```python
from build123d import *

# Parameters (mm, degrees)
SKETCH_1_W          = 30
SKETCH_1_H          = 30
SKETCH_1_W_2        = 26
SKETCH_1_H_2        = 26
EXTRUDE_1_DEPTH     = 580
SKETCH_2_W          = 50
SKETCH_2_H          = 20
CUT_EXTRUDE_1_DEPTH = 581.969018107
SKETCH_3_R          = 2.1
CUT_EXTRUDE_2_DEPTH = 581.969018107
SKETCH_4_R          = 2.1
CUT_EXTRUDE_3_DEPTH = 581.969018107
SKETCH_7_R          = 1.65
CUT_EXTRUDE_6_DEPTH = 581.969018107
SKETCH_8_R          = 1.65
CUT_EXTRUDE_7_DEPTH = 581.969018107
SKETCH_9_R          = 1.65
CUT_EXTRUDE_8_DEPTH = 581.969018107


with BuildPart() as part:
    # 草图1 → 凸台-拉伸1 (new body)
    with BuildSketch(Plane.XY):
        Rectangle(SKETCH_1_W, SKETCH_1_H)
        Rectangle(SKETCH_1_W_2, SKETCH_1_H_2, mode=Mode.SUBTRACT)
    extrude(amount=EXTRUDE_1_DEPTH)

    # 草图2 → 切除-拉伸1 (cut, through all)
    with BuildSketch(Plane.ZY.offset(15)):
        with Locations((115, 0)):
            Rectangle(SKETCH_2_W, SKETCH_2_H)
        with Locations((465, 0)):
            Rectangle(SKETCH_2_W, SKETCH_2_H)
    extrude(amount=-CUT_EXTRUDE_1_DEPTH, mode=Mode.SUBTRACT)

    # 草图3 → 切除-拉伸2 (cut, through all)
    with BuildSketch(Plane(origin=(0, 15, 0), x_dir=(1, 0, 0), z_dir=(0, 1, 0))):
        with Locations(Location((7.5, -10, 0), (0, 0, 270))):
            Circle(SKETCH_3_R)
        with Locations(Location((-7.5, -10, 0), (0, 0, 270))):
            Circle(SKETCH_3_R)
        with Locations(Location((-7.5, -570, 0), (0, 0, 270))):
            Circle(SKETCH_3_R)
        with Locations(Location((7.5, -570, 0), (0, 0, 270))):
            Circle(SKETCH_3_R)
    extrude(amount=-CUT_EXTRUDE_2_DEPTH, mode=Mode.SUBTRACT)

    # 草图4 → 切除-拉伸3 (cut, through all)
    with BuildSketch(Plane(origin=(0, 15, 0), x_dir=(1, 0, 0), z_dir=(0, 1, 0))):
        with Locations(Location((7.5, -401.567476668, 0), (0, 0, 270))):
            Circle(SKETCH_4_R)
        with Locations(Location((-7.5, -401.567476668, 0), (0, 0, 270))):
            Circle(SKETCH_4_R)
        with Locations(Location((-7.5, -381.567476668, 0), (0, 0, 270))):
            Circle(SKETCH_4_R)
        with Locations(Location((7.5, -381.567476668, 0), (0, 0, 270))):
            Circle(SKETCH_4_R)
        with Locations(Location((7.5, -178.432523332, 0), (0, 0, 270))):
            Circle(SKETCH_4_R)
        with Locations(Location((-7.5, -178.432523332, 0), (0, 0, 270))):
            Circle(SKETCH_4_R)
        with Locations(Location((-7.5, -198.432523332, 0), (0, 0, 270))):
            Circle(SKETCH_4_R)
        with Locations(Location((7.5, -198.432523332, 0), (0, 0, 270))):
            Circle(SKETCH_4_R)
        with Locations((162.5, -178.432523332)):
            Circle(SKETCH_4_R)
        with Locations((177.5, -178.432523332)):
            Circle(SKETCH_4_R)
        with Locations((177.5, -198.432523332)):
            Circle(SKETCH_4_R)
        with Locations((162.5, -198.432523332)):
            Circle(SKETCH_4_R)
        with Locations((162.5, -381.567476668)):
            Circle(SKETCH_4_R)
        with Locations((162.5, -401.567476668)):
            Circle(SKETCH_4_R)
        with Locations((177.5, -401.567476668)):
            Circle(SKETCH_4_R)
        with Locations((177.5, -381.567476668)):
            Circle(SKETCH_4_R)
    extrude(amount=-CUT_EXTRUDE_3_DEPTH, mode=Mode.SUBTRACT)

    # 草图7 → 切除-拉伸6 (cut, through all)
    with BuildSketch(Plane(origin=(0, 15, 0), x_dir=(1, 0, 0), z_dir=(0, 1, 0))):
        with Locations(Location((0, -33.5, 0), (0, 0, 270))):
            Circle(SKETCH_7_R)
        with Locations(Location((0, -58.5, 0), (0, 0, 270))):
            Circle(SKETCH_7_R)
        with Locations((167, -73.072466057)):
            Circle(SKETCH_7_R)
        with Locations((167, -48.072466057)):
            Circle(SKETCH_7_R)
    extrude(amount=-CUT_EXTRUDE_6_DEPTH, mode=Mode.SUBTRACT)

    # 草图8 → 切除-拉伸7 (cut, through all)
    with BuildSketch(Plane(origin=(0, 15, 0), x_dir=(1, 0, 0), z_dir=(0, 1, 0))):
        with Locations(Location((3, -506.927533943, 0), (0, 0, 270))):
            Circle(SKETCH_8_R)
        with Locations(Location((7, -521.975679885, 0), (0, 0, 270))):
            Circle(SKETCH_8_R)
        with Locations(Location((3, -531.927533943, 0), (0, 0, 270))):
            Circle(SKETCH_8_R)
        with Locations(Location((7, -546.975679885, 0), (0, 0, 270))):
            Circle(SKETCH_8_R)
    extrude(amount=-CUT_EXTRUDE_7_DEPTH, mode=Mode.SUBTRACT)

    # 草图9 → 切除-拉伸8 (cut, through all)
    with BuildSketch(Plane(origin=(0, 15, 0), x_dir=(1, 0, 0), z_dir=(0, 1, 0))):
        with Locations(Location((-7.5, -445, 0), (0, 0, 270))):
            Circle(SKETCH_9_R)
        with Locations(Location((7.5, -445, 0), (0, 0, 270))):
            Circle(SKETCH_9_R)
        with Locations(Location((7.5, -485, 0), (0, 0, 270))):
            Circle(SKETCH_9_R)
        with Locations(Location((-7.5, -485, 0), (0, 0, 270))):
            Circle(SKETCH_9_R)
        with Locations(Location((-7.5, -95, 0), (0, 0, 270))):
            Circle(SKETCH_9_R)
        with Locations(Location((7.5, -95, 0), (0, 0, 270))):
            Circle(SKETCH_9_R)
        with Locations(Location((-7.5, -135, 0), (0, 0, 270))):
            Circle(SKETCH_9_R)
        with Locations(Location((7.5, -135, 0), (0, 0, 270))):
            Circle(SKETCH_9_R)
    extrude(amount=-CUT_EXTRUDE_8_DEPTH, mode=Mode.SUBTRACT)


solid = part.part
```
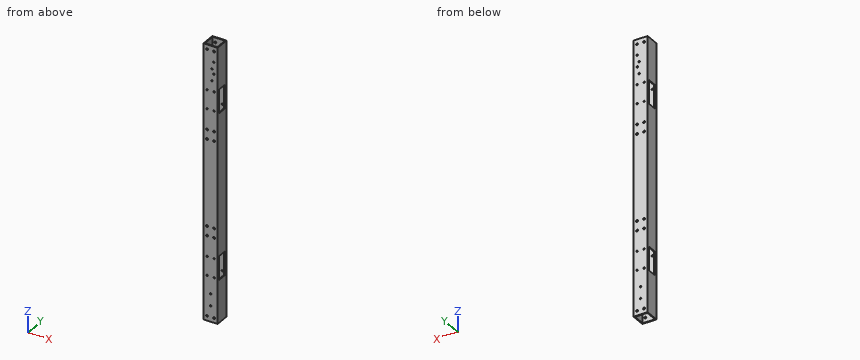
Part model, mm, in its own coordinate system. Round coordinates to 2 decimals unless told otherwise and drop trailing zeros. Write each loop counter-clockwise with the first axis right and the second up, starting at its lowest first coordinate (ties: lowest second). Pieces come first, ordered by that corner, then holes. Notation, with made-up numbers: (-15.5, 31) -> (-5.5, 31) arc R12 cw to (-5.5, 47) -> close; hole circle Ø6 at (89.25, 71.25). An arc over 180 degrees is marked (long way). Return JSON: item names as keys, results as strings. Group by question number.
Q1. Saw through at C-C on z = 351. Write the cut outline in (x, y), plus the area to 3 significant figures.
Q2. Saw through at A-A on z = 127. Write the cut outline in (x, y), plus the area to 3 significant figures.
Q3. Probe L1, parallel to X at y = -13.55, z = 95; L2, parallel to X at y = 11.5, z = 220. List the from-to ranges inside material, lowest first. Write a range as [from, to].
Q4. Pin check, flat tip, straight feed: pin 1 (3 mm diameter, centred on x = 7, z = 546.98, fed in from +Y). Stop position of the tip, or through.
Q5. Saw through at B-B on y = -1.25. Write the cut outline in (x, z), plus the area to 3 significant figures.
Answer:
{
 "1": {"outline": "(-15, -15) -> (15, -15) -> (15, 15) -> (-15, 15) -> close; hole (-13, -13) -> (13, -13) -> (13, 13) -> (-13, 13) -> close", "area": "224 mm2"},
 "2": {"outline": "(-15, -15) -> (15, -15) -> (15, -10) -> (13, -10) -> (13, -13) -> (-13, -13) -> (-13, -10) -> (-15, -10) -> close; (-15, 10) -> (-13, 10) -> (-13, 13) -> (13, 13) -> (13, 10) -> (15, 10) -> (15, 15) -> (-15, 15) -> close", "area": "144 mm2"},
 "3": {"L1": "[-15, -9.15], [-5.85, 5.85], [9.15, 15]", "L2": "[-15, -13], [13, 15]"},
 "4": {"pin 1": "through"},
 "5": {"outline": "(-15, 0) -> (-13, 0) -> (-13, 90) -> (-15, 90) -> close; (-15, 140) -> (-13, 140) -> (-13, 440) -> (-15, 440) -> close; (-15, 490) -> (-13, 490) -> (-13, 580) -> (-15, 580) -> close; (13, 0) -> (15, 0) -> (15, 90) -> (13, 90) -> close; (13, 140) -> (15, 140) -> (15, 440) -> (13, 440) -> close; (13, 490) -> (15, 490) -> (15, 580) -> (13, 580) -> close", "area": "1,920 mm2"}
}
